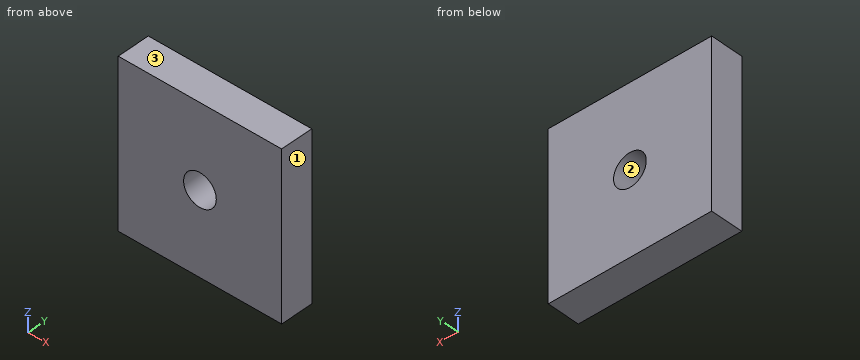
Autodesk Inventor part; units mm, degrees
ref_plane "YZ Plane" through (0, 0, 0) normal (1, 0, 0) x (0, 1, 0)
ref_plane "XZ Plane" through (0, 0, 0) normal (0, 1, 0) x (-1, 0, 0)
ref_plane "XY Plane" through (0, 0, 0) normal (0, 0, 1) x (1, 0, 0)
sketch "Sketch1" plane through (0, 0, 0) normal (0, 1, 0) x (-1, 0, 0)
  line L0 (50, 50) -> (-50, 50)
  line L1 (-50, 50) -> (-50, -50)
  line L2 (-50, -50) -> (50, -50)
  line L3 (50, -50) -> (50, 50)
  line L4 (50, 50) -> (-50, -50) construction
  line L5 (-50, 50) -> (50, -50) construction
  point P0 (0, 0)
  dimension "d0" = 100
  dimension "d1" = 100
extrude "Extrusion1" add sketch "Sketch1" along normal blind 20
sketch "Sketch2" plane through (0, 20, 0) normal (0, 1, 0) x (1, 0, 0)
  circle A0 centre (0, 0) radius 10
  dimension "d4" = 20
extrude "Extrusion2" cut sketch "Sketch2" against normal blind 20
properties part number "End"
Design review of the part built by this model. Coordinates are the model's own, in mm. Face numbers are marked on the shaded views. Coordinates: 2 decimals unless noted, no trailing zeros. Order: outer loops, then holes, each group sorted by start corner. A loop starts at its lowest first (then second) coordinate and runs counter-clockwise, first axis right, second up. Notation, with made-up numbers: M -11,27.25 L 43,27.25 A33 cw 43,57.25 Z; hole C 9,73 d9. An arc over 180 degrees is marked long. Use a Markdown table: item, result.
(1) Add section B-B (z = 0). Give the boundary of the cut face in (x, y).
Worked answers:
| item | result |
|---|---|
| outline | M -50,0 L -10,0 L -10,20 L -50,20 Z; M 10,0 L 50,0 L 50,20 L 10,20 Z |
(2) Add section C-C (y = 15.5). Give the boundary of the cut face in (x, z), then the cut area to 3 significant figures.
Worked answers:
| item | result |
|---|---|
| outline | M -50,-50 L 50,-50 L 50,50 L -50,50 Z; hole C 0,0 d20 |
| area | 9,690 mm2 |
(3) Add section A-A (x = 0). Give the boundary of the cut face in (y, z), then the cut area to 3 significant figures.
Worked answers:
| item | result |
|---|---|
| outline | M 0,-50 L 20,-50 L 20,-10 L 0,-10 Z; M 0,10 L 20,10 L 20,50 L 0,50 Z |
| area | 1,600 mm2 |
(4) Wall thickness on probe 1 along X at (y, z) = (7, 0): over which ranges is the line inside the solid? List them lowest first.
Worked answers:
| item | result |
|---|---|
| probe 1 | x = -50 to -10, 10 to 50 |
(5) Draft analysis for pull direction X (two halves, no side actions). For the marked faces 1, 2 and 3, state which applies: released by +X, released by -X, zero draft, split by the parting line, or undercut.
Worked answers:
| item | result |
|---|---|
| face 1 | released by +X |
| face 2 | undercut |
| face 3 | zero draft |
